```python
from build123d import *

# Parameters (mm, degrees)
BOSS_EXTRUDE2_DEPTH = 3.175


with BuildPart() as part:
    # sun → Boss-Extrude2 (new body)
    with BuildSketch(Plane(origin=(6.251367358, 48.255911881, 0), x_dir=(1, 0, 0), z_dir=(0, 0, 1))):
        Polygon((44.40620191, 170.247646781), (44.76575291, 170.284335781), (45.20263291, 170.222528781), (46.01571591, 169.872008781), (46.01571591, 169.332963781), (45.20263291, 168.982443781), (44.76575291, 168.920637781), (44.40620191, 168.957326781), (44.24731091, 168.056755781), (44.59783091, 167.968419781), (44.98729791, 167.760986781), (45.63132891, 167.153361781), (45.44703791, 166.647055781), (44.56311791, 166.595690781), (44.13159991, 166.686848781), (43.80619791, 166.844610781), (43.34899791, 166.052695781), (43.64815291, 165.849777781), (43.94307591, 165.521552781), (44.34044391, 164.730201781), (43.99415791, 164.317592781), (43.14579791, 164.571592781), (42.77157091, 164.804990781), (42.51982891, 165.064352781), (41.81907091, 164.476483781), (42.03101991, 164.183537781), (42.19583791, 163.774315781), (42.29856691, 162.894910781), (41.83205291, 162.625388781), (41.12169991, 163.154272781), (40.84991991, 163.501688781), (40.70203591, 163.831606781), (39.84266891, 163.518621781), (39.94144691, 163.170923781), (39.95640391, 162.730092781), (39.75207591, 161.868468781), (39.22149791, 161.775052781), (38.73494691, 162.514757781), (38.59835091, 162.934139781), (38.57210391, 163.294819781), (37.65770391, 163.294819781), (37.63145791, 162.934139781), (37.49486191, 162.514757781), (37.00831091, 161.775052781), (36.47773291, 161.868468781), (36.27340391, 162.730092781), (36.28836191, 163.170923781), (36.38713991, 163.518621781), (35.52777291, 163.831606781), (35.37988891, 163.501688781), (35.10810891, 163.154272781), (34.39775591, 162.625388781), (33.93124191, 162.894910781), (34.03397091, 163.774315781), (34.19878891, 164.183537781), (34.41073791, 164.476483781), (33.70997991, 165.064352781), (33.45823791, 164.804990781), (33.08401091, 164.571592781), (32.23565091, 164.317592781), (31.88936391, 164.730201781), (32.28673291, 165.521552781), (32.58165591, 165.849777781), (32.88081091, 166.052695781), (32.42361091, 166.844610781), (32.09820891, 166.686848781), (31.66669091, 166.595690781), (30.78277091, 166.647055781), (30.59847991, 167.153361781), (31.24251091, 167.760986781), (31.63197791, 167.968419781), (31.98249791, 168.056755781), (31.82360691, 168.957326781), (31.46405591, 168.920637781), (31.02717591, 168.982443781), (30.21409291, 169.332963781), (30.21409291, 169.872008781), (31.02717591, 170.222528781), (31.46405591, 170.284335781), (31.82360691, 170.247646781), (31.98249791, 171.148217781), (31.63197791, 171.236552781), (31.24251091, 171.443986781), (30.59847991, 172.051610781), (30.78277091, 172.557917781), (31.66669091, 172.609281781), (32.09820891, 172.518123781), (32.42361091, 172.360361781), (32.88081091, 173.152277781), (32.58165591, 173.355195781), (32.28673291, 173.683419781), (31.88936391, 174.474770781), (32.23565091, 174.887379781), (33.08401091, 174.633379781), (33.45823791, 174.399981781), (33.70997991, 174.140619781), (34.41073791, 174.728488781), (34.19878891, 175.021435781), (34.03397091, 175.430657781), (33.93124191, 176.310061781), (34.39775591, 176.579583781), (35.10810891, 176.050699781), (35.37988891, 175.703283781), (35.52777291, 175.373366781), (36.38713991, 175.686350781), (36.28836191, 176.034048781), (36.27340391, 176.474879781), (36.47773291, 177.336503781), (37.00831091, 177.429919781), (37.49486191, 176.690215781), (37.63145791, 176.270832781), (37.65770391, 175.910152781), (38.57210391, 175.910152781), (38.59835091, 176.270832781), (38.73494691, 176.690215781), (39.22149791, 177.429919781), (39.75207591, 177.336503781), (39.95640391, 176.474879781), (39.94144691, 176.034048781), (39.84266891, 175.686350781), (40.70203591, 175.373366781), (40.84991991, 175.703283781), (41.12169991, 176.050699781), (41.83205291, 176.579583781), (42.29856691, 176.310061781), (42.19583791, 175.430657781), (42.03101991, 175.021435781), (41.81907091, 174.728488781), (42.51982891, 174.140619781), (42.77157091, 174.399981781), (43.14579791, 174.633379781), (43.99415791, 174.887379781), (44.34044391, 174.474770781), (43.94307591, 173.683419781), (43.64815291, 173.355195781), (43.34899791, 173.152277781), (43.80619791, 172.360361781), (44.13159991, 172.518123781), (44.56311791, 172.609281781), (45.44703791, 172.557917781), (45.63132891, 172.051610781), (44.98729791, 171.443986781), (44.59783091, 171.236552781), (44.24731091, 171.148217781), align=None)
        with BuildLine():
            Line((35.44702391, 167.446136781), (40.78278491, 167.446136781))
            add(Edge.make_bspline(
                [(40.78278491, 167.446136781), (41.26046891, 168.035989781), (41.55007691, 168.788751781), (41.55007691, 169.606900781)],
                knots=[0, 0, 0, 0, 1, 1, 1, 1], degree=3))
            add(Edge.make_bspline(
                [(41.55007691, 169.606900781), (41.55007691, 170.425048781), (41.26046891, 171.168991781), (40.78278491, 171.758844781)],
                knots=[0, 0, 0, 0, 1, 1, 1, 1], degree=3))
            Line((40.78278491, 171.758844781), (35.44702391, 171.758844781))
            add(Edge.make_bspline(
                [(35.44702391, 171.758844781), (34.96933991, 171.168991781), (34.67973191, 170.425048781), (34.67973191, 169.606900781)],
                knots=[0, 0, 0, 0, 1, 1, 1, 1], degree=3))
            add(Edge.make_bspline(
                [(34.67973191, 169.606900781), (34.67973191, 168.788751781), (34.96933991, 168.035989781), (35.44702391, 167.446136781)],
                knots=[0, 0, 0, 0, 1, 1, 1, 1], degree=3))
        make_face(mode=Mode.SUBTRACT)
    extrude(amount=BOSS_EXTRUDE2_DEPTH)


solid = part.part
```
For this review, take the finished solid that the model builds, in its own axes (mm). A direction names the side the tool comes from. Round coordinates to 2 decimals unless told otherwise and drop trailing zeros. Write each loop counter-clockwise with the first axis right and the second up, starting at its lowest first coordinate (ties: lowest second). Pieces come first, ordered by that corner, then holes.
1) Machinability: for faces 1 (the face through (49.83, 212.7, 1.57)), 2 (the face through (51.855, 218.306, 1.565)), 3 (the face through (44, 215.702, 2)), 4 (the face through (44.4, 224.166, 1.6)), which of the approach directions +Z, -Z, +X, -X, +Y, -Y give a long, thin tool a straight path to every point of the face, cutting with its end or side? Answer none if there is none.
Answer below:
face 1: +Z, -Z, -Y
face 2: +Z, -Z, +X
face 3: +Z, -Z
face 4: +Z, -Z, +Y
2) Take a section at A-A on x = 45.25. Give the boundary of the cut face in (y, z) (3 decimals).
Answer below:
outline: (210.37, 0) - (215.702, 0) - (215.702, 3.175) - (210.37, 3.175) - close; (220.015, 0) - (225.347, 0) - (225.347, 3.175) - (220.015, 3.175) - close
3) Insertion check: pin 1 Ø1 at (x, z) = (48, 0.5) entering from -Y; pin 2 Ø1.6 at (x, z) = (44.5, 1.5) entering from +Y. Each pin has a flat end and moves straight along its axis. Give the tip position at first contact, or say it passes through.
Answer below:
pin 1: stops at y = 210.88
pin 2: stops at y = 225.42
4) For line 1 along Y through (x, z) = (44.25, 2.1); line 2 along X through (y, z) = (211.75, 3); line 3 along Y through (x, z) = (45.25, 0.3), list the stretches that pass through material, from the lowest coordinate up.
Answer below:
line 1: y = 211.55 to 215.7, 220.01 to 224.17
line 2: x = 40.25 to 41.63, 42.63 to 46.1, 47.11 to 48.48
line 3: y = 210.37 to 215.7, 220.01 to 225.35
5) Mouldability with a two-part tool opening along X and no side actions: class faces 5 (the face through (42.203, 223.784, 1.565)), 6 (the face through (40.233, 211.584, 1.565)), 7 (the face through (48.5, 224.13, 1.57)) as +X half, -X half, draft (parallel to the pull), parting line (faces both ways), or undercut.
Answer below:
face 5: undercut
face 6: -X half
face 7: +X half
